```python
from build123d import *

# Parameters (mm, degrees)
F2_DEPTH = 330


# Not quite as in the source:
# - a feature of the source that left no trace in its solid (it failed there, or was rolled back) is left out


with BuildPart() as f2:
    # F0 (on Front) → F2 (new body)
    with BuildSketch(Plane.XZ):
        Polygon((-166.6411012411, 147.3953723907), (-166.6411012411, 163.9132797718), (-193.8388049603, 163.9132797718), (-193.8388049603, -308.0049455166), (-185.2051019669, -308.0049455166), (-185.2051019669, -324.4089782238), (-166.6411012411, -324.4089782238), align=None)
    extrude(amount=F2_DEPTH)


solid = f2.part
```
Design review of the part built by this model. Coordinates are the model's own, in mm. A direction names the side the tool comes from. Coordinates: 2 decimals unless noted, no trailing zeros. Answer as a JSON object with one key per item and string values. Group by question number.
1) Wall thickness on L1, parallel to Z at x = -191.5, y = -232: over which ranges is the line inside the solid? List them lowest first.
2) Tool access review of faces 1 (the flat face through (-180, -163, 163.913)), 2 (the flat face through (-185.205, -163, -316)): name each direction out of +Z, -Z, +X, -X, +Y, -Y from which nothing blocks a thin tool from reaching the whole face with its end or side.
3) For pin 1 (7 mm diameter, centred on x = -190.5, y = -191, fed in from -Z); pin 2 (13 mm diameter, centred on y = -216, z = -315, fed in from -X), all flat-tipped, find the tip position at first contact; note any pin that passes through.
Computed values:
{
 "1": {"L1": "z = -308 to 163.91"},
 "2": {"face 1": "+Z, +X, -X, +Y, -Y", "face 2": "-Z, -X, +Y, -Y"},
 "3": {"pin 1": "stops at z = -308", "pin 2": "stops at x = -185.21"}
}
